Could you check a few things on this model? Use its own coordinates, in mm. Face numbers are marked on the shaded views. A direction names the side the tool comes from. Coordinates: 2 decimals unless noted, no trailing zeros. Write each loop counter-clockwise with the first axis right and the second up, starting at its lowest first coordinate (ties: lowest second). Pieces come first, ordered by that corner, then holes. Notation, with made-up numbers: (-17, 0) - (5, 0) arc R21 cw to (5, 37) - close; hole circle Ø3 at (-19.5, 54.25). An arc over 180 degrees is marked (long way). Write item = value, one per line. Start each with the question number.
```python
from build123d import *

# Parameters (mm, degrees)
SKETCH1_W                      = 96
SKETCH1_H                      = 64
BOSS_EXTRUDE1_DEPTH            = 1
SKETCH2_W                      = 96
SKETCH2_H                      = 64
SKETCH2_W_2                    = 72
SKETCH2_H_2                    = 52
BOSS_EXTRUDE2_DEPTH            = 21
SKETCH3_W                      = 72
SKETCH3_H                      = 3
BOSS_EXTRUDE3_DEPTH            = 4
SKETCH4_W                      = 72
SKETCH4_H                      = 6
CUT_EXTRUDE1_DEPTH             = 14
SKETCH5_W                      = 6
SKETCH5_H                      = 16
CUT_EXTRUDE2_DEPTH             = 60.363288319
CUT_EXTRUDE3_REACH             = 84.97
SKETCH6_W                      = 14
SKETCH6_H                      = 16
CUT_EXTRUDE3_DIRECTION_2_DEPTH = 83.969874051
SKETCH7_R                      = 1.6
CUT_EXTRUDE4_DEPTH             = 62.741396162
CUT_EXTRUDE5_DEPTH             = 8


with BuildPart() as part:
    # Sketch1 → Boss-Extrude1 (new body)
    with BuildSketch(Plane(origin=(0, 0, 0), x_dir=(1, 0, 0), z_dir=(0, 1, 0))):
        Rectangle(SKETCH1_W, SKETCH1_H)
    extrude(amount=BOSS_EXTRUDE1_DEPTH)

    # Sketch2 → Boss-Extrude2 (add)
    with BuildSketch(Plane(origin=(0, 1, 0), x_dir=(1, 0, 0), z_dir=(0, 1, 0))):
        Rectangle(SKETCH2_W, SKETCH2_H)
        with Locations((-4, 4)):
            Rectangle(SKETCH2_W_2, SKETCH2_H_2, mode=Mode.SUBTRACT)
    extrude(amount=BOSS_EXTRUDE2_DEPTH)

    # Sketch3 → Boss-Extrude3 (add)
    with BuildSketch(Plane(origin=(0, 1, 0), x_dir=(1, 0, 0), z_dir=(0, 1, 0))):
        with Locations((-4, -20.5)):
            Rectangle(SKETCH3_W, SKETCH3_H)
        with Locations((-4, 28.5)):
            Rectangle(SKETCH3_W, SKETCH3_H)
    extrude(amount=BOSS_EXTRUDE3_DEPTH)

    # Sketch4 → Cut-Extrude1 (cut)
    with BuildSketch(Plane(origin=(0, 22, 0), x_dir=(1, 0, 0), z_dir=(0, 1, 0))):
        Polygon((44, 30), (44, -28), (32, -28), (32, -22), (32, 30), align=None)
        with Locations((-4, -25)):
            Rectangle(SKETCH4_W, SKETCH4_H)
    extrude(amount=-CUT_EXTRUDE1_DEPTH, mode=Mode.SUBTRACT)

    # Sketch5 → Cut-Extrude2 (cut, through all)
    with BuildSketch(Plane(origin=(0, 8, 0), x_dir=(1, 0, 0), z_dir=(0, 1, 0))):
        with Locations((41, -20)):
            Rectangle(SKETCH5_W, SKETCH5_H)
    extrude(amount=-CUT_EXTRUDE2_DEPTH, mode=Mode.SUBTRACT)

    # Sketch6 → Cut-Extrude3 (cut, up to next)
    with BuildSketch(Plane(origin=(0, 0, -32), x_dir=(-1, 0, 0), z_dir=(0, 0, -1)), mode=Mode.PRIVATE) as cut_extrude3_sk1:
        with Locations((5, 14)):
            Rectangle(SKETCH6_W, SKETCH6_H)
    cut_extrude3_tool1 = extrude(cut_extrude3_sk1.sketch, amount=-CUT_EXTRUDE3_REACH, mode=Mode.PRIVATE) & part.part
    add(cut_extrude3_tool1.solids().sort_by_distance((-5, 14, -32))[0], mode=Mode.SUBTRACT)

    # Sketch6 → Cut-Extrude3 direction 2 (cut)
    with BuildSketch(Plane(origin=(0, 0, -32), x_dir=(-1, 0, 0), z_dir=(0, 0, -1))):
        with Locations((5, 14)):
            Rectangle(SKETCH6_W, SKETCH6_H)
    extrude(amount=CUT_EXTRUDE3_DIRECTION_2_DEPTH, mode=Mode.SUBTRACT)

    # Sketch7 → Cut-Extrude4 (cut, through all)
    with BuildSketch(Plane(origin=(0, 22, 0), x_dir=(1, 0, 0), z_dir=(0, 1, 0))):
        with Locations(Location((-42, 26, 0), (0, 0, 270))):
            Circle(SKETCH7_R)
        with Locations(Location((-42, -26, 0), (0, 0, 90))):
            Circle(SKETCH7_R)
        with Locations(Location((42, 26, 0), (0, 0, 270))):
            Circle(SKETCH7_R)
        with Locations(Location((42, -4, 0), (0, 0, 270))):
            Circle(SKETCH7_R)
    extrude(amount=-CUT_EXTRUDE4_DEPTH, mode=Mode.SUBTRACT)

    # Sketch9 → Cut-Extrude5 (cut)
    with BuildSketch(Plane.ZY.offset(48)):
        with BuildLine():
            Line((-18.285714286, 17), (-18.285714286, 5))
            ThreePointArc((-18.285714286, 5), (-20.285714286, 3), (-22.285714286, 5))
            Line((-22.285714286, 5), (-22.285714286, 17))
            ThreePointArc((-22.285714286, 17), (-20.285714286, 19), (-18.285714286, 17))
        make_face()
        with BuildLine():
            Line((-10.571428571, 17), (-10.571428571, 5))
            ThreePointArc((-10.571428571, 5), (-12.571428571, 3), (-14.571428571, 5))
            Line((-14.571428571, 5), (-14.571428571, 17))
            ThreePointArc((-14.571428571, 17), (-12.571428571, 19), (-10.571428571, 17))
        make_face()
        with BuildLine():
            Line((-2.857142857, 17), (-2.857142857, 5))
            ThreePointArc((-2.857142857, 5), (-4.857142857, 3), (-6.857142857, 5))
            Line((-6.857142857, 5), (-6.857142857, 17))
            ThreePointArc((-6.857142857, 17), (-4.857142857, 19), (-2.857142857, 17))
        make_face()
        with BuildLine():
            Line((4.857142857, 17), (4.857142857, 5))
            ThreePointArc((4.857142857, 5), (2.857142857, 3), (0.857142857, 5))
            Line((0.857142857, 5), (0.857142857, 17))
            ThreePointArc((0.857142857, 17), (2.857142857, 19), (4.857142857, 17))
        make_face()
        with BuildLine():
            Line((12.571428571, 17), (12.571428571, 5))
            ThreePointArc((12.571428571, 5), (10.571428571, 3), (8.571428571, 5))
            Line((8.571428571, 5), (8.571428571, 17))
            ThreePointArc((8.571428571, 17), (10.571428571, 19), (12.571428571, 17))
        make_face()
        with BuildLine():
            Line((20.285714286, 17), (20.285714286, 5))
            ThreePointArc((20.285714286, 5), (18.285714286, 3), (16.285714286, 5))
            Line((16.285714286, 5), (16.285714286, 17))
            ThreePointArc((16.285714286, 17), (18.285714286, 19), (20.285714286, 17))
        make_face()
    extrude(amount=-CUT_EXTRUDE5_DEPTH, mode=Mode.SUBTRACT)


solid = part.part
```
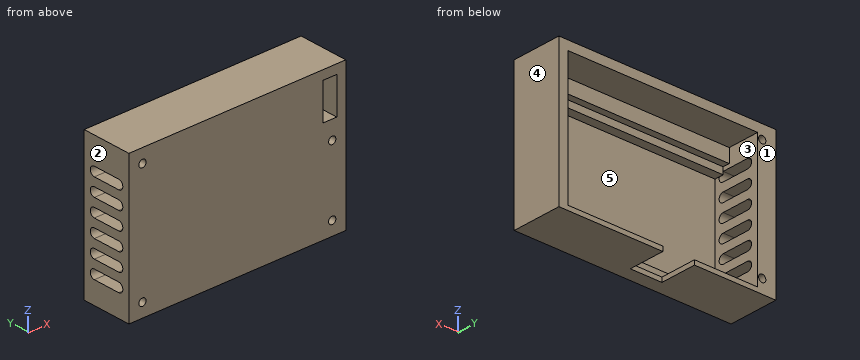
1) Suppose I cut it at D-D on z = 14. Please give me the cut outline in (x, y), plus the area to 3 significant figures.
2) Which directions (+Z, -Z, +X, -X, +Y, -Y) give clear straight access to the entire face, cutting with the end or side of a thin tool? Please do the marked faces 4 and 5.
3) Suppose I cut it at C-C on x = -38.5. Please give me the cut outline in (y, z).
4) Suppose I cut it at A-A on x = 42. Please give me the cut outline in (y, z), plus the area to 3 significant figures.
5) If I drill on probe 1 along X at (y, z) = (2.5, -26); probe 2 along Z at (x, y) = (-36.5, 12.75); probe 3 along X at (y, z) = (1.5, 20.5), over which ranges is the centre line in solid material (lowest first)? Write a range as [from, to].
6) Thinking about a two-plate mould opening in X: for the marked faces 1, 2 and 3, which applies, +X half, -X half, draft (parallel to the pull), parting line (faces both ways), or undercut?
7) For P1, Ø3, axis at x = -42, z = -26, coming from the -Y side; P2, Ø17.5, axis at x = -17, z = 1, coming from the +Y side, each with a flat end and sliding along its axis, tell me the tip position at first contact or that it passes through.
8) Suppose I cut it at B-B on z = 23. Please give me the cut outline in (x, y), plus the area to 3 significant figures.
Reply:
q1.outline = (-48, 0) - (38, 0) - (38, 8) - (32, 8) - (32, 1) - (-40, 1) - (-40, 22) - (-48, 22) - close; (44, 0) - (48, 0) - (48, 22) - (44, 22) - close
q1.area = 384 mm^2
q2.face_4 = +Z, -Z, +X, +Y, -Y
q2.face_5 = +Y
q3.outline = (0, -32) - (22, -32) - (22, -30) - (5, -30) - (5, -27) - (1, -27) - (1, 19) - (5, 19) - (5, 22) - (8, 22) - (8, 28) - (22, 28) - (22, 32) - (0, 32) - close
q4.outline = (0, -32) - (22, -32) - (22, -30) - (8, -30) - (8, -27.6) - (0, -27.6) - close; (0, -24.4) - (8, -24.4) - (8, 2.4) - (0, 2.4) - close; (0, 5.6) - (8, 5.6) - (8, 12) - (0, 12) - close; (0, 28) - (22, 28) - (22, 32) - (0, 32) - close
q4.area = 417 mm^2
q5.probe_1 = [-48, -43.6], [-40.4, -40], [32, 40.4], [43.6, 48]
q5.probe_2 = [-32, -30], [28, 32]
q5.probe_3 = [-48, 38], [44, 48]
q6.face_1 = draft
q6.face_2 = -X half
q6.face_3 = undercut
q7.P1 = through
q7.P2 = 1
q8.outline = (-48, 0) - (38, 0) - (38, 8) - (-40, 8) - (-40, 22) - (-48, 22) - close; (44, 0) - (48, 0) - (48, 22) - (44, 22) - close
q8.area = 888 mm^2
